from build123d import *

# Parameters (mm, degrees)
F1_DEPTH    = 2
F2_SIZE2    = 1.85
F2_SIZE     = 10
F2_2_SIZE2  = 1.85
F2_2_SIZE   = 10
F3_T1_DEPTH = 63.0781913019
F3_T3_DEPTH = 63.0781913019


# Not quite as in the source:
# - a fillet or chamfer that OpenCascade refuses, or shapes differently, is made with other operations: its cross-section is extruded or revolved along the edge and cut away or added


with BuildPart() as f1:
    # F0 (on Top) → F1 (new body, symmetric)
    with BuildSketch(Plane.XY):
        Polygon((-78.3224657339, 21.585099696), (-72.0955598013, 12.517264094), (48.031361701, 0), (51.9027564591, -13.106621107), (55.166546928, -13.106621107), (60.0622307678, 0), (86.172547065, -13.106621107), (119.6195638295, 0), (121.5894543095, 18.9048403295), (81.5894543095, 26.893378893), align=None)
    extrude(amount=F1_DEPTH, both=True)

    # F2
    f2_edges = [f1.edges().sort_by_distance(p)[0] for p in [
        (-12.032099, 6.258632, 2),
    ]]
    f2_side = f1.faces().sort_by_distance((40.734375, 11.652616, 2))[0]
    chamfer(f2_edges, length=F2_SIZE, length2=F2_SIZE2, reference=f2_side)

    # F2#2
    f2_2_edges = [f1.edges().sort_by_distance(p)[0] for p in [
        (-12.032099, 6.258632, -2),
    ]]
    f2_2_side = f1.faces().sort_by_distance((40.734375, 11.652616, -2))[0]
    chamfer(f2_2_edges, length=F2_2_SIZE, length2=F2_2_SIZE2, reference=f2_2_side)

    # F3: chamfer of 1.85 x 10 on 2 edges, made by hand

    # F3_s2 → F3_t1 (cut)
    with BuildSketch(Plane(origin=(-49.185702612, 71.6259198522, -12.2363892176), x_dir=(0.8243486911, 0.5660823575, 0), z_dir=(0.5605509501, -0.8162936645, 0.1394535249))):
        Polygon((-52.3460779882, 8.8318101599), (-42.4159004982, 5.802159781), (-52.3460779882, 6.9818101599), align=None)
    extrude(amount=F3_T1_DEPTH, mode=Mode.SUBTRACT)

    # F3_s4 → F3_t3 (cut)
    with BuildSketch(Plane(origin=(-49.185702612, 71.6259198522, 12.2363892176), x_dir=(0.8243486911, 0.5660823575, 0), z_dir=(0.5605509501, -0.8162936645, -0.1394535249))):
        Polygon((-52.3460779882, -8.8318101599), (-42.4159004982, -5.802159781), (-52.3460779882, -6.9818101599), align=None)
    extrude(amount=F3_T3_DEPTH, mode=Mode.SUBTRACT)


solid = f1.part
Could you check a few things on this model? Use its own coordinates, in mm. Give positions to 0.01 mm unless a question says otherwise; leave off trailing zeros. Loops run counter-clockwise (first coordinate to the right, second up) from the corner with the lowest first, then second, coordinate; pieces in that order, holes last. Notation, with made-up numbers: (-4.75, 73.25) -> (25.25, 73.25) arc R10 cw to (25.25, 79.25) -> close; hole circle Ø7 at (28.25, 67). An arc over 180 degrees is marked (long way). Answer as CSV lines item,"result". Start each with the question number.
(1) I need wall thicknesses on probe 1 along Y at (x, z) = (90.5, 1.25); probe 2 along Z at (x, y) = (-48.5, 12); probe 3 along Z at (x, y) = (-4, 12). Which ranges of each line are inside material? Lowest first, please.
(2) If we section it at D-D on x = -5: Write out the boundary of the cut face in (y, z), then the cut area to 3 significant figures.
(3) If we section it at C-C on x = 38: Write out the boundary of the cut face in (y, z), then the cut area to 3 significant figures.
(4) We'd pull the mould along X, two halves only. Please class faces 1 (the flat face through (57.58, -6.65, 0.03)), 2 (the flat face through (120.59, 9.32, 0.03)), 3 (the flat face through (72.93, -6.46, 0.03)), 4 (the flat face through (68, 12, -2)): released by +X, released by -X, zero draft, split by the parting line, or undercut.
(5) If we section it at B-B on z = 0.9: Write out the boundary of the cut face in (x, y), then the cut area to 3 significant figures.
(6) If we section it at A-A on y = -2.5: Write out the boundary of the cut face in (x, z).
Computed:
1,probe 1,"y = -11.41 to 25.11"
1,probe 2,"z = -0.51 to 0.51"
1,probe 3,"z = -1.36 to 1.36"
2,outline,"(5.53, -0.15) -> (15.58, -2) -> (24.02, -2) -> (24.02, 2) -> (15.58, 2) -> (5.53, 0.15) -> close"
2,area,"55.4 mm2"
3,outline,"(1.05, -0.15) -> (11.1, -2) -> (25.45, -2) -> (25.45, 2) -> (11.1, 2) -> (1.05, 0.15) -> close"
3,area,"79.0 mm2"
4,face 1,"undercut"
4,face 2,"released by +X"
4,face 3,"undercut"
4,face 4,"zero draft"
5,outline,"(-72.51, 21.78) -> (-62.14, 15.56) -> (46.79, 4.21) -> (51.9, -13.11) -> (55.17, -13.11) -> (60.06, 0) -> (86.17, -13.11) -> (119.62, 0) -> (121.59, 18.9) -> (81.59, 26.89) -> close"
5,area,"3,870 mm2"
6,outline,"(48.77, -2) -> (59.13, -2) -> (59.13, 2) -> (48.77, 2) -> close; (65.04, -2) -> (113.24, -2) -> (113.24, 2) -> (65.04, 2) -> close"
